The listing builds one solid part. Answer for the finished solid, in the listing's coordinates (mm). Face numbers are marked on the shaded views. A direction names the side the tool comes from. Give positions to 0.01 mm unless a question says otherwise; leave off trailing zeros. Loops run counter-clockwise (first coordinate to the right, second up) from the corner with the lowest first, then second, coordinate; pieces in that order, holes last. Notation, with made-up numbers: M 59,-39 L 84,-39 A25 cw 84,-3 Z; hole C 65,72.5 d10. An arc over 180 degrees is marked long. One line per item, written item: value. Start each with the question number.
Q1. A cutting plane is placed at D-D, the plane z = 2.75. Determine the outline of the cut face in (x, y), and give its area (3 significant figures).
Q2. Consider L1, parallel to X at y = 35.85, z = 12.5; L2, parallel to Y at x = 15, z = 2.65; L3, parallel to X at y = -25, z = 3.6. Determine where each line is inside the solid, lowest interval first.
Q3. A cutting plane is placed at A-A, the plane x = 0. Determine the outline of the cut face in (y, z).
Q4. A cutting plane is placed at C-C, the plane y = 5. Determine the outline of the cut face in (x, z), and give its area (3 significant figures).
Q5. A cutting plane is placed at B-B, the plane z = 12.5. Determine the outline of the cut face in (x, y), and give its area (3 significant figures).
Q6. For the marked faces 1 and 2, determine the directions among +Z, -Z, +X, -X, +Y, -Y from which every point of the face is accessible in a straight line to the end or side of a thin tool.
Q7. Flat-ended cylindrical pins translate along their axes: pin 1 (4.5 mm diameter, centred on x = 15, y = -25, fed in from -Z); pin 2 (4.5 mm diameter, centred on x = 15.5, z = 12.5, fed in from -Y); pin 3 (10 mm diameter, centred on x = 2, z = 9, fed in from -Y); pin 4 (8 mm diameter, centred on x = 14, z = 11, fed in from -Y). Find the tip coordinate at first contact, or state that the pin passes through.
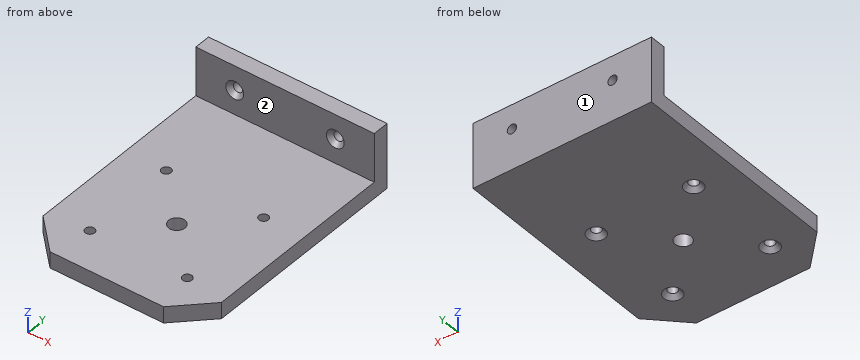
from build123d import *

# Parameters (mm, degrees)
BOSS_EXTRUDE1_DEPTH                               = 5
CUT_EXTRUDE1_REACH                                = 7
SKETCH2_R                                         = 2.5
SKETCH3_W                                         = 55
SKETCH3_H                                         = 5
BOSS_EXTRUDE2_DEPTH                               = 15
CSK_FOR_M2_5_FLAT_HEAD_MACHINE_SCREW1_D           = 2.9
CSK_FOR_M2_5_FLAT_HEAD_MACHINE_SCREW1_CSINK_D     = 5.5
CSK_FOR_M2_5_FLAT_HEAD_MACHINE_SCREW1_CSINK_ANGLE = 90
CSK_FOR_M2_5_FLAT_HEAD_MACHINE_SCREW2_D           = 2.9
CSK_FOR_M2_5_FLAT_HEAD_MACHINE_SCREW2_DEPTH       = 5
CSK_FOR_M2_5_FLAT_HEAD_MACHINE_SCREW2_CSINK_D     = 5.5
CSK_FOR_M2_5_FLAT_HEAD_MACHINE_SCREW2_CSINK_ANGLE = 90


with BuildPart() as part:
    # Sketch1 → Boss-Extrude1 (new body)
    with BuildSketch(Plane.XY):
        Polygon((-17.5, -37.5), (-27.5, -27.5), (-27.5, 37.5), (27.5, 37.5), (27.5, -27.5), (17.5, -37.5), align=None)
    extrude(amount=BOSS_EXTRUDE1_DEPTH)

    # Sketch2 → Cut-Extrude1 (cut, up to next)
    with BuildSketch(Plane.XY.offset(5), mode=Mode.PRIVATE) as cut_extrude1_sk1:
        with Locations((0, -10)):
            Circle(SKETCH2_R)
    cut_extrude1_tool1 = extrude(cut_extrude1_sk1.sketch, amount=-CUT_EXTRUDE1_REACH, mode=Mode.PRIVATE) & part.part
    add(cut_extrude1_tool1.solids().sort_by_distance((0, -10, 5))[0], mode=Mode.SUBTRACT)

    # Sketch3 → Boss-Extrude2 (add)
    with BuildSketch(Plane.XY.offset(5)):
        with Locations((0, 35)):
            Rectangle(SKETCH3_W, SKETCH3_H)
    extrude(amount=BOSS_EXTRUDE2_DEPTH)

    # CSK for M2.5 Flat Head Machine Screw1 (through all)
    with Locations(Plane(origin=(0, 32.5, 0), x_dir=(-1, 0, 0), z_dir=(0, -1, 0))):
        with Locations((-15.5, -12.5), (15.5, -12.5)):
            CounterSinkHole(CSK_FOR_M2_5_FLAT_HEAD_MACHINE_SCREW1_D / 2, CSK_FOR_M2_5_FLAT_HEAD_MACHINE_SCREW1_CSINK_D / 2, counter_sink_angle=CSK_FOR_M2_5_FLAT_HEAD_MACHINE_SCREW1_CSINK_ANGLE)

    # CSK for M2.5 Flat Head Machine Screw2
    with Locations(Plane(origin=(0, 0, 0), x_dir=(-1, 0, 0), z_dir=(0, 0, -1))):
        with Locations((-15, 5), (15, 5), (-15, -25), (15, -25)):
            CounterSinkHole(CSK_FOR_M2_5_FLAT_HEAD_MACHINE_SCREW2_D / 2, CSK_FOR_M2_5_FLAT_HEAD_MACHINE_SCREW2_CSINK_D / 2, depth=CSK_FOR_M2_5_FLAT_HEAD_MACHINE_SCREW2_DEPTH, counter_sink_angle=CSK_FOR_M2_5_FLAT_HEAD_MACHINE_SCREW2_CSINK_ANGLE)


solid = part.part
Answer block:
1. outline: M -27.5,-27.5 L -17.5,-37.5 L 17.5,-37.5 L 27.5,-27.5 L 27.5,37.5 L -27.5,37.5 Z; hole C -15,-25 d2.9; hole C -15,5 d2.9; hole C 0,-10 d5; hole C 15,-25 d2.9; hole C 15,5 d2.9
1. area: 3,980 mm^2
2. L1: -27.5 to -16.95, -14.05 to 14.05, 16.95 to 27.5
2. L2: -37.5 to -26.45, -23.55 to 3.55, 6.45 to 37.5
2. L3: -27.5 to -16.45, -13.55 to 13.55, 16.45 to 27.5
3. outline: M -37.5,0 L -12.5,0 L -12.5,5 L -37.5,5 Z; M -7.5,0 L 37.5,0 L 37.5,20 L 32.5,20 L 32.5,5 L -7.5,5 Z
4. outline: M -27.5,0 L -17.75,0 L -16.45,1.3 L -16.45,5 L -27.5,5 Z; M -13.55,1.3 L -12.25,0 L 12.25,0 L 13.55,1.3 L 13.55,5 L -13.55,5 Z; M 16.45,1.3 L 17.75,0 L 27.5,0 L 27.5,5 L 16.45,5 Z
4. area: 243 mm^2
5. outline: M -27.5,32.5 L -18.25,32.5 L -16.95,33.8 L -16.95,37.5 L -27.5,37.5 Z; M -14.05,33.8 L -12.75,32.5 L 12.75,32.5 L 14.05,33.8 L 14.05,37.5 L -14.05,37.5 Z; M 16.95,33.8 L 18.25,32.5 L 27.5,32.5 L 27.5,37.5 L 16.95,37.5 Z
5. area: 243 mm^2
6. face 1: +Z, -Z, +X, -X, +Y
6. face 2: +Z, +X, -X, -Y
7. pin 1: z = 0.5
7. pin 2: y = 33
7. pin 3: y = -37.5
7. pin 4: y = 32.5
